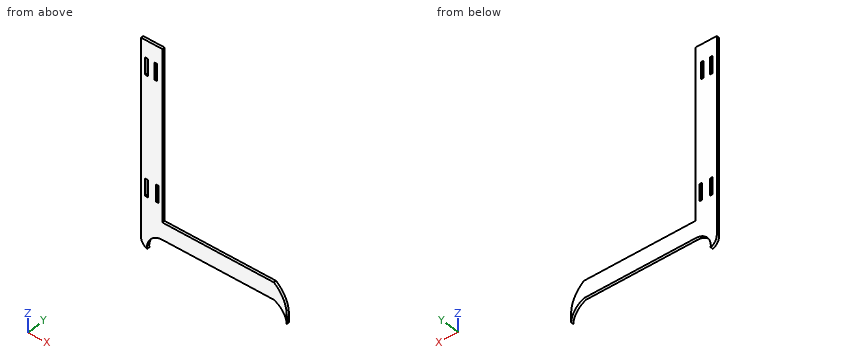
from build123d import *

# Parameters (mm, degrees)
F0_W     = 3
F0_H     = 20
F0_W_2   = 3.000302
F1_DEPTH = 3


with BuildPart() as f1:
    # F0 (on Front) → F1 (new body)
    with BuildSketch(Plane.XZ):
        with BuildLine():
            Line((12.508355, -100.066841), (12.508355, 100.066841))
            Line((12.508355, 100.066841), (-12.491645, 100.066841))
            Line((-12.491645, 100.066841), (-12.491645, -100.066841))
            Line((-12.491645, -100.066841), (-12.491645, -130.066841))
            ThreePointArc((-12.491645, -130.066841), (-10.550096, -136.186191), (-5.435743, -140.066841))
            ThreePointArc((-5.435743, -140.066841), (-0.926587, -126.062712), (12.508355, -120.066841))
            Line((12.508355, -120.066841), (20.482657, -120.066841))
            Line((20.482657, -120.066841), (142.29022, -120.066841))
            ThreePointArc((142.29022, -120.066841), (152.807868, -127.853683), (157.508355, -140.066841))
            Line((157.508355, -140.066841), (157.508355, -130.066841))
            ThreePointArc((157.508355, -130.066841), (153.549375, -113.296332), (142.508355, -100.066841))
            Line((142.508355, -100.066841), (12.508355, -100.066841))
        make_face()
        with Locations((-6.187321, -70.066841)):
            Rectangle(F0_W, F0_H, mode=Mode.SUBTRACT)
        Polygon((4.798322, -60.066841), (6.254178, -60.066841), (7.798322, -60.066841), (7.798322, -80.066841), (4.798322, -80.066841), align=None, mode=Mode.SUBTRACT)
        Polygon((-4.687321, 59.832168), (-6.230536, 59.832168), (-6.254178, 59.832168), (-7.687321, 59.832168), (-7.687321, 79.832168), (-4.687321, 79.832168), align=None, mode=Mode.SUBTRACT)
        with Locations((4.62724, 69.832168)):
            Rectangle(F0_W_2, F0_H, mode=Mode.SUBTRACT)
    extrude(amount=F1_DEPTH)


solid = f1.part
Build history of the part. All positions in model axes, mm. Give positions to 0.01 mm unless a question says otherwise; leave off trailing zeros. Loops run counter-clockwise (first coordinate to the right, second up) from the corner with the lowest first, then second, coordinate; pieces in that order, holes last. Notation, with made-up numbers: (-20, 46) -> (-8, 46) arc R37 cw to (-8, 82) -> close; hole circle Ø8 at (39.25, 69.5). An arc over 180 degrees is marked (long way). Answer in a Markdown table with one row per item.
Item 1: Slice it at C-C on z = -9.5. Write the cut outline in (x, y), plus the area to 3 significant figures.
Findings below:
| item | result |
|---|---|
| outline | (-12.49, -3) -> (12.51, -3) -> (12.51, 0) -> (-12.49, 0) -> close |
| area | 75.0 mm² |
Item 2: Flat gauge pins, fed straight in: P1, Ø1.5, axis at y = -1.5, z = 71, coming from the +X side; P2, Ø0.9, axis at x = 73.5, y = -1, coming from the +Z side; P3, Ø1.5, axis at x = -7, y = -2, coming from the -Z side. Where does each tip first touch, or does it go through?
Findings below:
| item | result |
|---|---|
| P1 | stops at x = 12.51 |
| P2 | stops at z = -100.07 |
| P3 | stops at z = -139.74 |
Item 3: Probe line 1 along X through (y, z) = (-1.95, 60); line 2 along X through (y, z) = (-1.15, -13); line 3 along Z through (x, y) = (99.5, -0.45). List the from-to ranges inside material, lowest first. Write a range as [from, to].
Findings below:
| item | result |
|---|---|
| line 1 | x = [-12.49, -7.69], [-4.69, 3.13], [6.13, 12.51] |
| line 2 | x = [-12.49, 12.51] |
| line 3 | z = [-120.07, -100.07] |
Item 4: Slice it at B-B on x = 134. Write the cut outline in (y, z).
Findings below:
| item | result |
|---|---|
| outline | (-3, -120.07) -> (0, -120.07) -> (0, -100.07) -> (-3, -100.07) -> close |
Item 5: Slice it at A-A on y = -2.3. Write the cut outline in (x, z).
Findings below:
| item | result |
|---|---|
| outline | (-12.49, -130.07) arc R10.61 ccw to (-5.44, -140.07) arc R18.05 cw to (12.51, -120.07) -> (142.29, -120.07) arc R23.43 cw to (157.51, -140.07) -> (157.51, -130.07) arc R37.5 ccw to (142.51, -100.07) -> (12.51, -100.07) -> (12.51, 100.07) -> (-12.49, 100.07) -> close; hole (-7.69, -80.07) -> (-4.69, -80.07) -> (-4.69, -60.07) -> (-7.69, -60.07) -> close; hole (-7.69, 59.83) -> (-4.69, 59.83) -> (-4.69, 79.83) -> (-7.69, 79.83) -> close; hole (3.13, 59.83) -> (6.13, 59.83) -> (6.13, 79.83) -> (3.13, 79.83) -> close; hole (4.8, -80.07) -> (7.8, -80.07) -> (7.8, -60.07) -> (4.8, -60.07) -> close |
